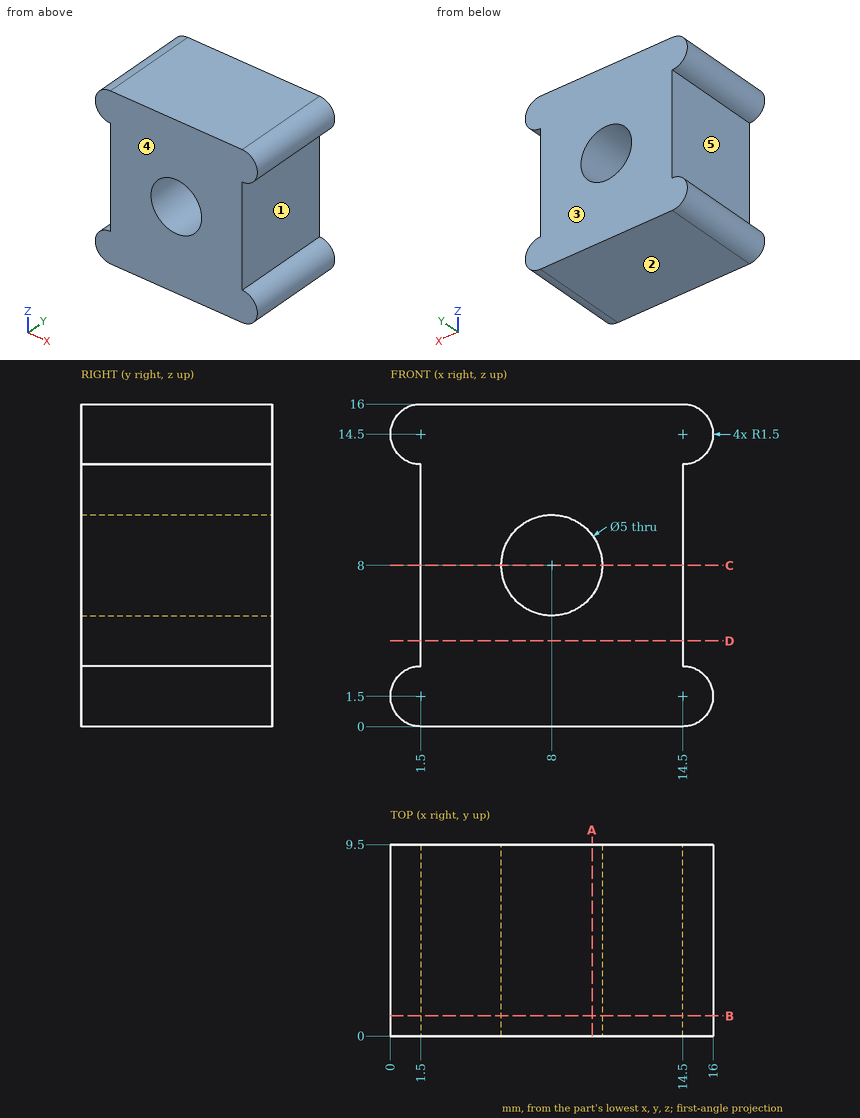
Verification items for this drawing (mm, ordinates from the low corner). A direction names the side the tool comes from. Give positions to 0.01 mm unless a question says otherwise; leave off trailing zeros. Loops run counter-clockwise (first coordinate to the right, second up) from the corner with the lowest first, then second, coordinate; pieces in that order, holes last. Notation, with made-up numbers: M 39,-29 L 92,-29 A18 cw 92,-19 Z; hole C -0.5,43 d3. An arc over 180 degrees is marked long. Answer as a JSON object with one key per item and string values. Group by question number.
Item 1: Sectioned sample at C-C on z = 8. Record the boundary of the cut face in (x, y), plus the area to 3 significant figures.
Item 2: Mould release check, pull along Z, two halves, no side actions. Record for the marked faces 1, 2 and 3: pulls with the +Z half, pulls with the -Z half, needs draft (parallel to the pull), parting line crosses it, or undercut.
Item 3: Sectioned sample at A-A on x = 10. Record the boundary of the cut face in (y, z).
Item 4: Sectioned sample at B-B on y = 1. Record the boundary of the cut face in (x, z), plus the area to 3 significant figures.
Item 5: Access from +Z, -Z, +X, -X, +Y, -Y to the whole of each face (thin tool, end or side, straight path). Record for the marked faces 4 and 5.
Item 6: Sectioned sample at D-D on z = 4.25. Record the boundary of the cut face in (x, y), plus the area to 4 significant figures.
Item 7: Material ranges on L1, parallel to Z at x = 8, y = 2.5; L2, parallel to X at y = 7.25, z = 8; L3, parallel to X at y = 8, z = 12.25, recorded low to high.
Item 8: Gauge pin test, flat ends, axial feed: pin 1 (1 mm diameter, centred on y = 3.5, z = 10, fed in from +X); pin 2 (4 mm diameter, centred on y = 6.5, z = 10.5, fed in from -X). Record the tip position at first contact, or that the pin passes through.
Findings below:
{
 "1": {"outline": "M 1.5,0 L 5.5,0 L 5.5,9.5 L 1.5,9.5 Z; M 10.5,0 L 14.5,0 L 14.5,9.5 L 10.5,9.5 Z", "area": "76.0 mm2"},
 "2": {"face 1": "undercut", "face 2": "pulls with the -Z half", "face 3": "needs draft"},
 "3": {"outline": "M 0,0 L 9.5,0 L 9.5,6.5 L 0,6.5 Z; M 0,9.5 L 9.5,9.5 L 9.5,16 L 0,16 Z"},
 "4": {"outline": "M 1.5,0 L 14.5,0 A1.5 ccw 14.5,3 L 14.5,13 A1.5 ccw 14.5,16 L 1.5,16 A1.5 ccw 1.5,13 L 1.5,3 A1.5 ccw Z; hole C 8,8 d5", "area": "203 mm2"},
 "5": {"face 4": "+Z, -Z, +X, -X, -Y", "face 5": "-X, +Y, -Y"},
 "6": {"outline": "M 1.5,0 L 14.5,0 L 14.5,9.5 L 1.5,9.5 Z", "area": "123.5 mm2"},
 "7": {"L1": "0 to 5.5, 10.5 to 16", "L2": "1.5 to 5.5, 10.5 to 14.5", "L3": "1.5 to 14.5"},
 "8": {"pin 1": "x = 14.5", "pin 2": "x = 1.5"}
}
